Geometry: final body of the model. Coordinates: model frame, mm. A direction names the side the tool comes from. Give positions to 0.01 mm unless a question says otherwise; leave off trailing zeros. Loops run counter-clockwise (first coordinate to the right, second up) from the corner with the lowest first, then second, coordinate; pieces in that order, holes last. Notation, with made-up numbers: (51.5, -7) -> (86.5, -7) arc R22 cw to (86.5, 27) -> close; hole circle Ø6 at (59.25, 1). An arc over 180 degrees is marked (long way). One line per question, with ' | ' between items. Start each with the question number.
Item 1: Material intervals for line 1 along Y through (x, z) = (-10, -1.75); line 2 along Z through (x, y) = (6, -16); line 3 along Y through (x, z) = (0, -4), sorted ascending. Write a range as [from, to].
Item 2: Set-up query: faces 1 (the flat face through (0, -13, 2.54)), 2 (the cylindrical face through (-0.382, -21.089, -3.633)), 3 (the flat face through (0, -26, -1.575)). Return all of +Z, -Z, +X, -X, +Y, -Y with unobstructed straight access to the full face (end or side cutting, diameter ignored); none if empty.
Item 3: Section A-A on y = -9.5. Return loops of the section in (x, z) (3 decimals), then the cut area to 3 significant figures.
Item 4: Section B-B on x = 3.5. Return loops of the section in (y, z), then the cut area to 3 significant figures.
Item 5: Pin query (flat end, axial travel): P1, Ø1.3, axis at y = -26.5, z = 0, coming from the +X side; P2, Ø5, axis at x = -5, y = -13.5, coming from the +Z side; P3, Ø2, axis at x = -6.5, y = -26.5, coming from the +Z side. Return the tip coordinate at first contact, or that it passes through.
Item 6: Mould query, pull axis X, two halves, no side actions, for faces 4 (the flat face through (0, -27.889, 0)), 5 (the cylindrical face through (-37.014, -13.128, -5.204)), 6 (the cylindrical face through (-0.382, -4.311, -3.633)). Classes: released by +X, released by -X, zero draft, split by the parting line, or undercut.
from build123d import *

# Parameters (mm, degrees)
F0_W          = 76.2
F0_H          = 12.7
F1_DEPTH      = 25.4
F2_W          = 50.292
F2_H          = 3.1496
F3_DEPTH      = 2.4892
F4_R          = 0.762
F5_R          = 0.508
F6_R          = 3.81
F7_W          = 64.77
F7_H          = 20.32
F8_DEPTH      = 3.81
F9_R          = 5.08
F10_T1_DEPTH  = 54.61
F10_T3_DEPTH  = 10.16
F10_T6_ANGLE  = 90
F10_T8_ANGLE  = 90
F10_T10_ANGLE = 90
F10_T12_ANGLE = 90
F11_W         = 64.77
F11_H         = 20.32
F12_DEPTH     = 3.81
F13_R         = 5.08
F14_T1_DEPTH  = 54.61
F14_T3_DEPTH  = 10.16
F14_T6_ANGLE  = 90
F14_T8_ANGLE  = 90
F14_T10_ANGLE = 90
F14_T12_ANGLE = 90
F15_R         = 0.508


# Not quite as in the source:
# - a fillet or chamfer that OpenCascade refuses, or shapes differently, is made with other operations: its cross-section is extruded or revolved along the edge and cut away or added


with BuildPart() as f1:
    # F0 (on Front) → F1 (new body)
    with BuildSketch(Plane.XZ):
        Rectangle(F0_W, F0_H)
    extrude(amount=F1_DEPTH)

    # F2 (on face) → F3 (join)
    with BuildSketch(Plane.XZ.offset(25.4)):
        Rectangle(F2_W, F2_H)
    extrude(amount=F3_DEPTH)

    # F4
    f4_edges = [f1.edges().sort_by_distance(p)[0] for p in [
        (-25.146, -26.6446, 1.5748),
        (-25.146, -26.6446, -1.5748),
        (25.146, -26.6446, 1.5748),
        (25.146, -26.6446, -1.5748),
    ]]
    fillet(f4_edges, radius=F4_R)

    # F5
    f5_edges = [f1.edges().sort_by_distance(p)[0] for p in [
        (0, -27.8892, 1.5748),
        (24.922815, -27.8892, 1.351615),
        (-24.922815, -27.8892, 1.351615),
        (25.146, -27.8892, 0),
        (-25.146, -27.8892, 0),
        (24.922815, -27.8892, -1.351615),
        (-24.922815, -27.8892, -1.351615),
        (0, -27.8892, -1.5748),
    ]]
    fillet(f5_edges, radius=F5_R)

    # F6
    f6_edges = [f1.edges().sort_by_distance(p)[0] for p in [
        (38.1, -12.7, 6.35),
        (38.1, -12.7, -6.35),
        (-38.1, -12.7, 6.35),
        (-38.1, -12.7, -6.35),
    ]]
    fillet(f6_edges, radius=F6_R)

    # F7 (on face) → F8 (cut)
    with BuildSketch(Plane.XY.offset(6.35)):
        with Locations((0, -12.7)):
            Rectangle(F7_W, F7_H)
    extrude(amount=-F8_DEPTH, mode=Mode.SUBTRACT)

    # F9
    f9_edges = [f1.edges().sort_by_distance(p)[0] for p in [
        (-32.385, -2.54, 4.445),
        (-32.385, -22.86, 4.445),
        (32.385, -2.54, 4.445),
        (32.385, -22.86, 4.445),
    ]]
    fillet(f9_edges, radius=F9_R)

    # F10: fillet of radius 5.08 on 1 edges, made by hand

    # F10_s2 → F10_t1 (join)
    with BuildSketch(Plane.YZ.offset(-27.305)):
        with BuildLine():
            ThreePointArc((-2.54, 6.35), (-4.3478368763, 3.6039073716), (-7.4586888497, 2.54))
            Line((-7.4586888497, 2.54), (-2.54, 2.54))
            Line((-2.54, 2.54), (-2.54, 6.35))
        make_face()
        with BuildLine():
            ThreePointArc((-22.86, 6.35), (-21.0521631237, 3.6039073716), (-17.9413111503, 2.54))
            Line((-17.9413111503, 2.54), (-22.86, 2.54))
            Line((-22.86, 2.54), (-22.86, 6.35))
        make_face()
    extrude(amount=F10_T1_DEPTH)

    # F10_s4 → F10_t3 (join)
    with BuildSketch(Plane.XZ.offset(7.62)):
        with BuildLine():
            ThreePointArc((-32.385, 6.35), (-30.5771631237, 3.6039073716), (-27.4663111503, 2.54))
            Line((-27.4663111503, 2.54), (-32.385, 2.54))
            Line((-32.385, 2.54), (-32.385, 6.35))
        make_face()
        with BuildLine():
            ThreePointArc((32.385, 6.35), (30.5771631237, 3.6039073716), (27.4663111503, 2.54))
            Line((27.4663111503, 2.54), (32.385, 2.54))
            Line((32.385, 2.54), (32.385, 6.35))
        make_face()
    extrude(amount=F10_T3_DEPTH)

    # F10_s5 → F10_t6 (revolve)
    with BuildSketch(Plane.XZ.offset(7.62)):
        with BuildLine():
            ThreePointArc((32.385, 6.35), (30.5771631237, 3.6039073716), (27.4663111503, 2.54))
            Line((27.4663111503, 2.54), (32.385, 2.54))
            Line((32.385, 2.54), (32.385, 6.35))
        make_face()
    revolve(axis=Axis((27.305, -7.62, 2.54), (0, 0, 1)), revolution_arc=F10_T6_ANGLE)

    # F10_s7 → F10_t8 (revolve)
    with BuildSketch(Plane.XZ.offset(7.62)):
        with BuildLine():
            ThreePointArc((-32.385, 6.35), (-30.5771631237, 3.6039073716), (-27.4663111503, 2.54))
            Line((-27.4663111503, 2.54), (-32.385, 2.54))
            Line((-32.385, 2.54), (-32.385, 6.35))
        make_face()
    revolve(axis=Axis((-27.305, -7.62, 2.54), (0, 0, -1)), revolution_arc=F10_T8_ANGLE)

    # F10_s9 → F10_t10 (revolve)
    with BuildSketch(Plane.YZ.offset(-27.305)):
        with BuildLine():
            ThreePointArc((-22.86, 6.35), (-21.0521631237, 3.6039073716), (-17.9413111503, 2.54))
            Line((-17.9413111503, 2.54), (-22.86, 2.54))
            Line((-22.86, 2.54), (-22.86, 6.35))
        make_face()
    revolve(axis=Axis((-27.305, -17.78, 2.54), (0, 0, -1)), revolution_arc=F10_T10_ANGLE)

    # F10_s11 → F10_t12 (revolve)
    with BuildSketch(Plane.XZ.offset(17.78)):
        with BuildLine():
            ThreePointArc((32.385, 6.35), (30.5771631237, 3.6039073716), (27.4663111503, 2.54))
            Line((27.4663111503, 2.54), (32.385, 2.54))
            Line((32.385, 2.54), (32.385, 6.35))
        make_face()
    revolve(axis=Axis((27.305, -17.78, 2.54), (0, 0, -1)), revolution_arc=F10_T12_ANGLE)

    # F11 (on face) → F12 (cut)
    with BuildSketch(Plane(origin=(0, 0, -6.35), x_dir=(1, 0, 0), z_dir=(0, 0, -1))):
        with Locations((0, 12.7)):
            Rectangle(F11_W, F11_H)
    extrude(amount=-F12_DEPTH, mode=Mode.SUBTRACT)

    # F13
    f13_edges = [f1.edges().sort_by_distance(p)[0] for p in [
        (32.385, -22.86, -4.445),
        (32.385, -2.54, -4.445),
        (-32.385, -22.86, -4.445),
        (-32.385, -2.54, -4.445),
    ]]
    fillet(f13_edges, radius=F13_R)

    # F14: fillet of radius 5.08 on 1 edges, made by hand

    # F14_s2 → F14_t1 (join)
    with BuildSketch(Plane.YZ.offset(-27.305)):
        with BuildLine():
            ThreePointArc((-22.86, -6.35), (-21.0521631237, -3.6039073716), (-17.9413111503, -2.54))
            Line((-17.9413111503, -2.54), (-22.86, -2.54))
            Line((-22.86, -2.54), (-22.86, -6.35))
        make_face()
        with BuildLine():
            ThreePointArc((-2.54, -6.35), (-4.3478368763, -3.6039073716), (-7.4586888497, -2.54))
            Line((-7.4586888497, -2.54), (-2.54, -2.54))
            Line((-2.54, -2.54), (-2.54, -6.35))
        make_face()
    extrude(amount=F14_T1_DEPTH)

    # F14_s4 → F14_t3 (join)
    with BuildSketch(Plane.XZ.offset(7.62)):
        with BuildLine():
            ThreePointArc((32.385, -6.35), (30.5771631237, -3.6039073716), (27.4663111503, -2.54))
            Line((27.4663111503, -2.54), (32.385, -2.54))
            Line((32.385, -2.54), (32.385, -6.35))
        make_face()
        with BuildLine():
            ThreePointArc((-32.385, -6.35), (-30.5771631237, -3.6039073716), (-27.4663111503, -2.54))
            Line((-27.4663111503, -2.54), (-32.385, -2.54))
            Line((-32.385, -2.54), (-32.385, -6.35))
        make_face()
    extrude(amount=F14_T3_DEPTH)

    # F14_s5 → F14_t6 (revolve)
    with BuildSketch(Plane.YZ.offset(27.305)):
        with BuildLine():
            ThreePointArc((-22.86, -6.35), (-21.0521631237, -3.6039073716), (-17.9413111503, -2.54))
            Line((-17.9413111503, -2.54), (-22.86, -2.54))
            Line((-22.86, -2.54), (-22.86, -6.35))
        make_face()
    revolve(axis=Axis((27.305, -17.78, -2.54), (0, 0, 1)), revolution_arc=F14_T6_ANGLE)

    # F14_s7 → F14_t8 (revolve)
    with BuildSketch(Plane.YZ.offset(27.305)):
        with BuildLine():
            ThreePointArc((-2.54, -6.35), (-4.3478368763, -3.6039073716), (-7.4586888497, -2.54))
            Line((-7.4586888497, -2.54), (-2.54, -2.54))
            Line((-2.54, -2.54), (-2.54, -6.35))
        make_face()
    revolve(axis=Axis((27.305, -7.62, -2.54), (0, 0, -1)), revolution_arc=F14_T8_ANGLE)

    # F14_s9 → F14_t10 (revolve)
    with BuildSketch(Plane.YZ.offset(-27.305)):
        with BuildLine():
            ThreePointArc((-2.54, -6.35), (-4.3478368763, -3.6039073716), (-7.4586888497, -2.54))
            Line((-7.4586888497, -2.54), (-2.54, -2.54))
            Line((-2.54, -2.54), (-2.54, -6.35))
        make_face()
    revolve(axis=Axis((-27.305, -7.62, -2.54), (0, 0, 1)), revolution_arc=F14_T10_ANGLE)

    # F14_s11 → F14_t12 (revolve)
    with BuildSketch(Plane.XZ.offset(17.78)):
        with BuildLine():
            ThreePointArc((-32.385, -6.35), (-30.5771631237, -3.6039073716), (-27.4663111503, -2.54))
            Line((-27.4663111503, -2.54), (-32.385, -2.54))
            Line((-32.385, -2.54), (-32.385, -6.35))
        make_face()
    revolve(axis=Axis((-27.305, -17.78, -2.54), (0, 0, 1)), revolution_arc=F14_T12_ANGLE)

    # F15
    f15_edges = [f1.edges().sort_by_distance(p)[0] for p in [
        (-36.984077, 0, 5.234077),
        (0, 0, -6.35),
        (0, 0, 6.35),
        (36.984077, 0, 5.234077),
        (38.1, 0, 0),
        (-38.1, 0, 0),
        (36.984077, 0, -5.234077),
        (-36.984077, 0, -5.234077),
    ]]
    fillet(f15_edges, radius=F15_R)


solid = f1.part
Result sheet:
1) line 1: y = [-25.4, 0] | line 2: z = [-2.54, 2.54] | line 3: y = [-25.4, -21.51], [-3.89, 0]
2) face 1: +Z | face 2: -Z | face 3: -Z, +X, -X, -Y
3) outline: (-38.1, -2.54) arc R3.81 ccw to (-34.29, -6.35) -> (-32.385, -6.35) arc R5.08 cw to (-27.466, -2.54) -> (27.466, -2.54) arc R5.08 cw to (32.385, -6.35) -> (34.29, -6.35) arc R3.81 ccw to (38.1, -2.54) -> (38.1, 2.54) arc R3.81 ccw to (34.29, 6.35) -> (32.385, 6.35) arc R5.08 cw to (27.466, 2.54) -> (-27.466, 2.54) arc R5.08 cw to (-32.385, 6.35) -> (-34.29, 6.35) arc R3.81 ccw to (-38.1, 2.54) -> close | area: 481 mm²
4) outline: (-27.89, -1.07) arc R0.51 ccw to (-27.38, -1.57) -> (-25.4, -1.57) -> (-25.4, -6.35) -> (-22.86, -6.35) arc R5.08 cw to (-17.94, -2.54) -> (-7.46, -2.54) arc R5.08 cw to (-2.54, -6.35) -> (-0.51, -6.35) arc R0.51 ccw to (0, -5.84) -> (0, 5.84) arc R0.51 ccw to (-0.51, 6.35) -> (-2.54, 6.35) arc R5.08 cw to (-7.46, 2.54) -> (-17.94, 2.54) arc R5.08 cw to (-22.86, 6.35) -> (-25.4, 6.35) -> (-25.4, 1.57) -> (-27.38, 1.57) arc R0.51 ccw to (-27.89, 1.07) -> close | area: 195 mm²
5) P1: stops at x = 25.15 | P2: stops at z = 2.54 | P3: stops at z = 1.57
6) face 4: zero draft | face 5: released by -X | face 6: undercut
